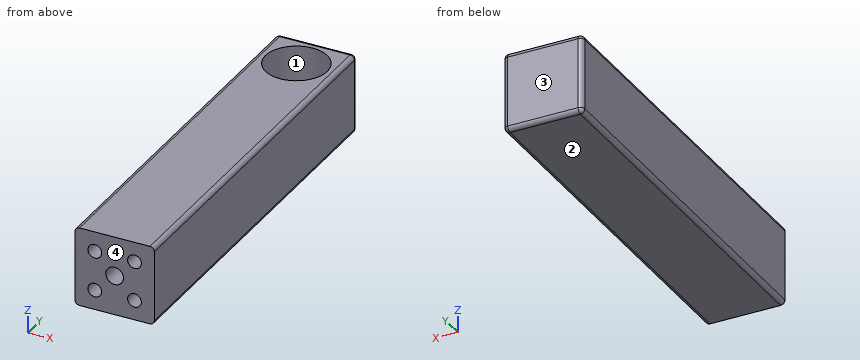
from build123d import *

# Parameters (mm, degrees)
BOSS_EXTRUDE1_DEPTH = 279.4
SKETCH1_4_R         = 4.96062
CUT_EXTRUDE1_DEPTH  = 25.4
SKETCH1_5_R         = 6.35
CUT_EXTRUDE2_DEPTH  = 250.825
FILLET1_R           = 3.175
SKETCH4_R           = 22.225
CUT_EXTRUDE3_DEPTH  = 44.45


with BuildPart() as part:
    # Sketch1 → Boss-Extrude1 (new body)
    with BuildSketch(Plane(origin=(0, 0, 0), x_dir=(1, 0, 0), z_dir=(0, 1, 0))):
        with BuildLine():
            Line((-24.257, 27.504571429), (26.543, 27.504571429))
            ThreePointArc((26.543, 27.504571429), (28.78806403, 26.574635459), (29.718, 24.329571429))
            Line((29.718, 24.329571429), (29.718, -26.470428571))
            ThreePointArc((29.718, -26.470428571), (28.78806403, -28.715492602), (26.543, -29.645428571))
            Line((26.543, -29.645428571), (-24.257, -29.645428571))
            ThreePointArc((-24.257, -29.645428571), (-26.50206403, -28.715492602), (-27.432, -26.470428571))
            Line((-27.432, -26.470428571), (-27.432, 24.329571429))
            ThreePointArc((-27.432, 24.329571429), (-26.50206403, 26.574635459), (-24.257, 27.504571429))
        make_face()
    extrude(amount=BOSS_EXTRUDE1_DEPTH)

    # Sketch1<4> → Cut-Extrude1 (cut)
    with BuildSketch(Plane(origin=(0, 0, 0), x_dir=(1, 0, 0), z_dir=(0, 1, 0))):
        with Locations((-13.1445, 13.217071429)):
            Circle(SKETCH1_4_R)
        with Locations((15.4305, 13.217071429)):
            Circle(SKETCH1_4_R)
        with Locations((15.4305, -15.357928571)):
            Circle(SKETCH1_4_R)
        with Locations((-13.1445, -15.357928571)):
            Circle(SKETCH1_4_R)
    extrude(amount=CUT_EXTRUDE1_DEPTH, mode=Mode.SUBTRACT)

    # Sketch1<5> → Cut-Extrude2 (cut)
    with BuildSketch(Plane(origin=(0, 0, 0), x_dir=(1, 0, 0), z_dir=(0, 1, 0))):
        with Locations((1.143, -1.070428571)):
            Circle(SKETCH1_5_R)
    extrude(amount=CUT_EXTRUDE2_DEPTH, mode=Mode.SUBTRACT)

    # Fillet1
    fillet1_edges = [part.edges().sort_by_distance(p)[0] for p in [
        (-26.50206403, 279.4, 28.715492602),
        (1.143, 279.4, 29.645428571),
        (28.78806403, 279.4, 28.715492602),
        (29.718, 279.4, 1.070428571),
        (28.78806403, 279.4, -26.574635459),
        (1.143, 279.4, -27.504571429),
        (-26.50206403, 279.4, -26.574635459),
        (-27.432, 279.4, 1.070428571),
    ]]
    fillet(fillet1_edges, radius=FILLET1_R)

    # Sketch4 → Cut-Extrude3 (cut)
    with BuildSketch(Plane.XY.offset(29.645428571)):
        with Locations((1.143, 250.825)):
            Circle(SKETCH4_R)
    extrude(amount=-CUT_EXTRUDE3_DEPTH, mode=Mode.SUBTRACT)


solid = part.part
Read the model definition and answer for the solid it produces. Units are mm, in the model's axes. Face numbers are marked on the shaded views. Coordinates: 2 decimals unless noted, no trailing zeros. Loops run counter-clockwise (first coordinate to the right, second up) from the corner with the lowest first, then second, coordinate; pieces in that order, holes last. Notation, with made-up numbers: (-4.75, 13) -> (2.25, 13) arc R32 cw to (2.25, 46) -> close; hole circle Ø2 at (-12.5, 82.25). An arc over 180 degrees is marked (long way). Write item = value, one per line. Start each with the question number.
1) The part is cut by section D-D, the plane y = 234. Determine the outline of the cut face in (x, z) (3 decimals), plus the area to 3 significant figures.
2) Given P1, Ø13.5, axis at x = 5, y = 251.5, coming from the +Z side; P2, Ø9, axis at x = 15.43, z = -13.22, coming from the -Y side, each flat-ended and moving along its own axis, determine where each tip first touches the part or whether it passes through.
3) Find the intervals of material crossed by L1, parallel to Z at x = 8, y = 261; L2, parallel to X at y = 218, z = -24.5; L3, parallel to X at y = 252.5, z = -11, in increasing order. Write a range as from..to.
4) The part is cut by section A-A, the plane x = -1. Determine the outline of the cut face in (y, z) (3 decimals).
5) The mould has two halves that part along Y. Classify the marked faces 1, 2, 3 and 4: pulls with the +Y half, pulls with the -Y half, needs draft (parallel to the pull), parting line crosses it, or undercut.
6) The part is cut by section B-B, the plane y = 44. Determine the outline of the cut face in (x, z) (3 decimals), plus the area to 3 significant figures.
Result:
q1.outline = (-27.432, -24.33) arc R3.175 ccw to (-24.257, -27.505) -> (26.543, -27.505) arc R3.175 ccw to (29.718, -24.33) -> (29.718, 26.47) arc R3.175 ccw to (26.543, 29.645) -> (15.664, 29.645) -> (15.664, -14.805) -> (-13.378, -14.805) -> (-13.378, 29.645) -> (-24.257, 29.645) arc R3.175 ccw to (-27.432, 26.47) -> close
q1.area = 1,970 mm²
q2.P1 = -14.8
q2.P2 = 25.4
q3.L1 = -27.5..-14.8
q3.L2 = -27.43..29.71
q3.L3 = -27.43..-21.02, 23.3..29.72
q4.outline = (0, -27.505) -> (276.225, -27.505) arc R3.175 ccw to (279.4, -24.33) -> (279.4, 26.47) arc R3.175 ccw to (276.225, 29.645) -> (272.946, 29.645) -> (272.946, -14.805) -> (228.704, -14.805) -> (228.704, -4.907) -> (0, -4.907) -> close; (0, 7.048) -> (228.704, 7.048) -> (228.704, 29.645) -> (0, 29.645) -> close
q5.face_1 = undercut
q5.face_2 = needs draft
q5.face_3 = pulls with the +Y half
q5.face_4 = pulls with the -Y half
q6.outline = (-27.432, -24.33) arc R3.175 ccw to (-24.257, -27.505) -> (26.543, -27.505) arc R3.175 ccw to (29.718, -24.33) -> (29.718, 26.47) arc R3.175 ccw to (26.543, 29.645) -> (-24.257, 29.645) arc R3.175 ccw to (-27.432, 26.47) -> close; hole circle Ø12.7 at (1.143, 1.07)
q6.area = 3,130 mm²
